Input: part model. Units: mm. Frame: model coordinates. Face numbers are marked on the shaded views. A direction names the side the tool comes from. Coordinates: 2 decimals unless noted, no trailing zeros. Write each loop counter-clockwise with the first axis right and the second up, starting at its lowest first coordinate (ties: lowest second). Pieces come first, ordered by that corner, then holes. Notation, with made-up numbers: M 30,43 L 71,43 A23 ccw 71,58 Z; hole C 3.5,-39.5 d6. An arc over 180 degrees is marked long. Write each question's results on one line, items separated by ' | '. Start each with the question number.
1. Section query C-C, the plane y = 36.5. Output: boundary loops of the cut face in (x, z).
2. Set-up query: the marked faces 1 and 2. Return all of +Z, -Z, +X, -X, +Y, -Y with unobstructed straight access to the full face (end or side cutting, diameter ignored); none if empty.
3. Section query B-B, the plane z = 20.5. Output: boundary loops of the cut face in (x, y).
4. Ray query, probe 1 along Z at (x, y) = (32.5, 1.4); probe 2 along X at (y, z) = (1, 5); probe 3 along X at (y, z) = (6, 11). Return the intervals inside material, ascending.
5. Section query D-D, the plane z = 12. Output: boundary loops of the cut face in (x, y).
6. Section query A-A, the plane x = 32.5. Output: boundary loops of the cut face in (y, z), and give its area (3 significant figures).
7. First-contact query: pin 1 (6.5 mm diameter, centred on x = 7.5, z = 35.5, fed in from +Y); pin 2 (1 mm diameter, centred on x = 1.5, y = 26.5, fed in from -Z); pin 3 (1.5 mm diameter, centred on y = 11.5, z = 26, fed in from +X). Flat tips, straight axial feed; report the tip coordinate or a pass-through.
```python
from build123d import *

# Parameters (mm, degrees)
BOSS_EXTRUDE1_DEPTH = 40
HOLE1_D             = 5
CUT_EXTRUDE1_DEPTH  = 40
CUT_EXTRUDE2_DEPTH  = 40
SKETCH7_R           = 1.5
CUT_EXTRUDE3_DEPTH  = 40
FILLET1_R           = 1
SKETCH10_R          = 2.5
CUT_EXTRUDE4_DEPTH  = 40


with BuildPart() as part:
    # Sketch2 → Boss-Extrude1 (new body)
    with BuildSketch(Plane.XY):
        with BuildLine():
            Line((2, 0), (40, 0))
            Line((40, 0), (40, 2))
            Line((40, 2), (3, 2))
            ThreePointArc((3, 2), (2.292893219, 2.292893219), (2, 3))
            Line((2, 3), (2, 45))
            Line((2, 45), (0, 45))
            Line((0, 45), (0, 2))
            ThreePointArc((0, 2), (0.585786438, 0.585786438), (2, 0))
        make_face()
    extrude(amount=BOSS_EXTRUDE1_DEPTH)

    # Hole1 (through all)
    with Locations(Plane(origin=(0, 2, 0), x_dir=(1, 0, 0), z_dir=(0, 1, 0))):
        with Locations((32.5, -35.5), (32.5, -5.5), (7.5, -5.5), (7.5, -35.5)):
            Hole(HOLE1_D / 2)

    # Sketch5 → Cut-Extrude1 (cut)
    with BuildSketch(Plane(origin=(2, 0, 0), x_dir=(0, 0, -1), z_dir=(1, 0, 0))):
        with BuildLine():
            Line((-40, 45), (-40, 24))
            ThreePointArc((-40, 24), (-20, 44), (0, 24))
            Line((0, 24), (0, 45))
            Line((0, 45), (-40, 45))
        make_face()
    extrude(amount=-CUT_EXTRUDE1_DEPTH, mode=Mode.SUBTRACT)

    # Sketch6 → Cut-Extrude2 (cut)
    with BuildSketch(Plane(origin=(2, 0, 0), x_dir=(0, 0, -1), z_dir=(1, 0, 0))):
        with BuildLine():
            Line((-14, 34.5), (-14, 18.5))
            ThreePointArc((-14, 18.5), (-20, 12.5), (-26, 18.5))
            Line((-26, 18.5), (-26, 34.5))
            ThreePointArc((-26, 34.5), (-20, 40.5), (-14, 34.5))
        make_face()
    extrude(amount=-CUT_EXTRUDE2_DEPTH, mode=Mode.SUBTRACT)

    # Sketch7 → Cut-Extrude3 (cut)
    with BuildSketch(Plane(origin=(2, 0, 0), x_dir=(0, 0, -1), z_dir=(1, 0, 0))):
        with Locations((-4.735, 26.5)):
            Circle(SKETCH7_R)
        with Locations((-35.265, 26.5)):
            Circle(SKETCH7_R)
        with Locations((-27.6325, 13.280122211)):
            Circle(SKETCH7_R)
        with Locations((-12.3675, 13.280122211)):
            Circle(SKETCH7_R)
        with Locations((-27.6325, 39.719877789)):
            Circle(SKETCH7_R)
        with Locations((-12.3675, 39.719877789)):
            Circle(SKETCH7_R)
    extrude(amount=-CUT_EXTRUDE3_DEPTH, mode=Mode.SUBTRACT)

    # Fillet1
    fillet1_edges = [part.edges().sort_by_distance(p)[0] for p in [
        (40, 1, 0),
        (40, 1, 40),
    ]]
    fillet(fillet1_edges, radius=FILLET1_R)

    # Sketch10 → Cut-Extrude4 (cut)
    with BuildSketch(Plane(origin=(0, 2, 0), x_dir=(1, 0, 0), z_dir=(0, 1, 0))):
        with Locations((7.5, -20.5)):
            Circle(SKETCH10_R)
        with Locations((32.5, -20.5)):
            Circle(SKETCH10_R)
    extrude(amount=-CUT_EXTRUDE4_DEPTH, mode=Mode.SUBTRACT)


solid = part.part
```
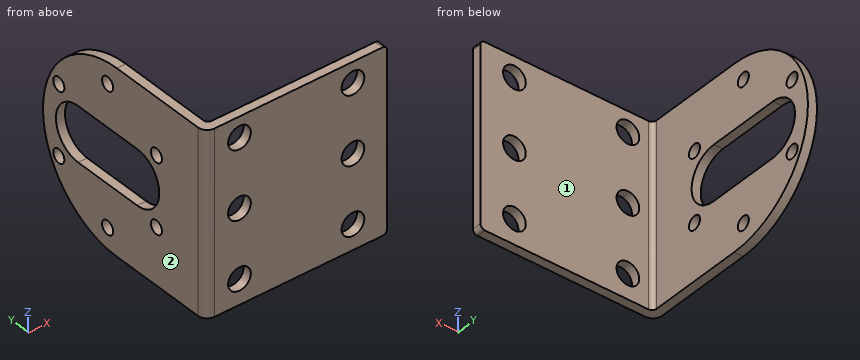
Answer:
1) outline: M 0,4.39 L 2,4.39 L 2,14.34 L 0,14.34 Z; M 0,25.66 L 2,25.66 L 2,35.61 L 0,35.61 Z
2) face 1: +Z, -Z, +X, +Y | face 2: +Z, -Z, -X, +Y, -Y
3) outline: M 0,2 A2 ccw 2,0 L 5,0 L 5,2 L 3,2 A1 cw 2,3 L 2,12.52 L 0,12.52 Z; M 0,40.48 L 2,40.48 L 2,43.99 L 0,43.99 Z; M 10,0 L 30,0 L 30,2 L 10,2 Z; M 35,0 L 40,0 L 40,2 L 35,2 Z
4) probe 1: 0 to 3, 8 to 18, 23 to 33, 38 to 40 | probe 2: 0.27 to 5.05, 9.95 to 30.05, 34.95 to 40 | probe 3: 0 to 2
5) outline: M 0,2 A2 ccw 2,0 L 40,0 L 40,2 L 3,2 A1 cw 2,3 L 2,11.83 L 0,11.83 Z; M 0,14.73 L 2,14.73 L 2,38.27 L 0,38.27 Z; M 0,41.17 L 2,41.17 L 2,42.33 L 0,42.33 Z
6) outline: M 0,0 L 2,0 L 2,3 L 0,3 Z; M 0,8 L 2,8 L 2,18 L 0,18 Z; M 0,23 L 2,23 L 2,33 L 0,33 Z; M 0,38 L 2,38 L 2,40 L 0,40 Z | area: 50.0 mm^2
7) pin 1: y = 2 | pin 2: z = 0.1 | pin 3: x = 2
